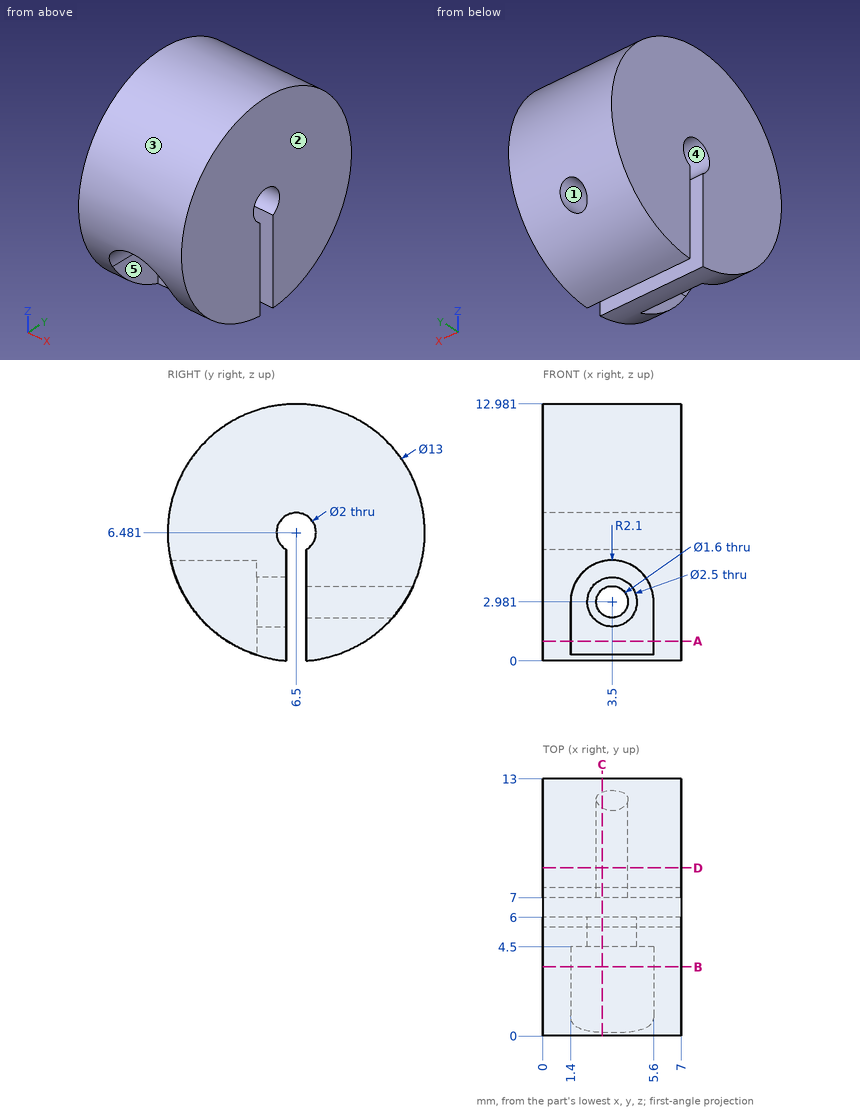
For this review, use the dimensioned drawing (mm, ordinates from the lowest corner) and the shaded views. A direction names the side the tool comes from. Round coordinates to 2 decimals unless told otherwise and drop trailing zeros. Order: outer loops, then holes, each group sorted by start corner. A loop starts at its lowest first (then second) coordinate and runs counter-clockwise, first axis right, second up. Notation, with made-up numbers: (89, -18.5) -> (121, -18.5) arc R31 cw to (121, 11.5) -> close; hole circle Ø6 at (80, 10.5). An arc over 180 degrees is marked (long way). Write item = value, one per line. Start each with the question number.
Item 1: Consider section B-B on y = 3.5. Write out the cut boundary in (x, z), plus the area to 3 significant figures.
Item 2: For the marked faces 4 and 5, list the 3-axis set-ups (+Z, -Z, +X, -X, +Y, -Y) from which the entire face can be reached by the end or side of a thin tool; tool diameter is ignored.
Item 3: Consider section D-D on y = 8.5. Write out the cut boundary in (x, z) (1 decimal), plus the area to 3 significant figures.
Item 4: Consider section A-A on z = 1. Write out the cut boundary in (x, y) (1 decimal).
Item 5: Consider section C-C on x = 3. Write out the cut boundary in (y, z) (1 decimal).
Item 6: For line 1 along Y through (x, z) = (5.75, 6.5); line 2 along Z through (x, y) = (4, 6.5); line 3 along Z through (x, y) = (1, 7.25) (1 decimal), list the stretches that pass through material, from the lowest coordinate up.
Item 7: Mouldability with a two-part tool opening along Z and no side actions: class the marked faces 1, 2 and 3 as released by +Z, released by -Z, zero draft, split by the parting line, or undercut.
Item 8: Clearance check with flat-ended pins moving along their axes: pin 1 Ø1.5 at (x, y) = (5, 5.5) entering from -Z; pin 2 Ø1.6 at (y, z) = (6.5, 6.48) entering from -X; pin 3 Ø4 at (x, y) = (2, 1.5) entering from +Z; pin 4 Ø1.5 at (x, y) = (3.5, 8.5) entering from +Z. State where each tip first meets the part, or that it passes through.
Conclusion:
q1.outline = (0, 0.71) -> (1.4, 0.71) -> (1.4, 2.98) arc R2.1 cw to (5.6, 2.98) -> (5.6, 0.71) -> (7, 0.71) -> (7, 12.25) -> (0, 12.25) -> close
q1.area = 64.3 mm2
q2.face_4 = +X, -X
q2.face_5 = -Z, -Y
q3.outline = (0, 0.3) -> (7, 0.3) -> (7, 12.7) -> (0, 12.7) -> close; hole circle Ø1.6 at (3.5, 3)
q3.area = 84.6 mm2
q4.outline = (0, 3) -> (1.4, 3) -> (1.4, 4.5) -> (5.6, 4.5) -> (5.6, 3) -> (7, 3) -> (7, 6) -> (0, 6) -> close; (0, 7) -> (7, 7) -> (7, 10) -> (0, 10) -> close
q5.outline = (0.2, 5) -> (4.5, 5) -> (4.5, 4.1) -> (6, 4.1) -> (6, 5.6) arc R1 cw (long way) to (7, 5.6) -> (7, 3.6) -> (12.3, 3.6) arc R6.5 ccw (long way) to start; (4.5, 0.3) arc R6.5 ccw to (6, 0) -> (6, 1.8) -> (4.5, 1.8) -> close; (7, 0) arc R6.5 ccw to (11.5, 2.4) -> (7, 2.4) -> close
q6.line_1 = 0 to 5.5, 7.5 to 13
q6.line_2 = 7.48 to 12.98
q6.line_3 = 0 to 5.8, 7.1 to 12.9
q7.face_1 = undercut
q7.face_2 = zero draft
q7.face_3 = split by the parting line
q8.pin_1 = 0
q8.pin_2 = through
q8.pin_3 = 12.25
q8.pin_4 = 12.86
